Part model, mm, in its own coordinate system. Face numbers are marked on the shaded views. A direction names the side the tool comes from. Coordinates: 2 decimals unless noted, no trailing zeros. Order: outer loops, then holes, each group sorted by start corner. A loop starts at its lowest first (then second) coordinate and runs counter-clockwise, first axis right, second up.
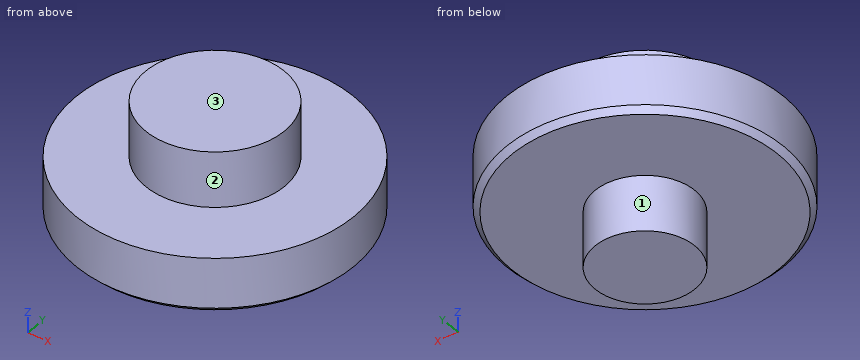
from build123d import *

# Parameters (mm, degrees)
SKETCH_R     = 50
PAD_DEPTH    = 20
CHAMFER_SIZE = 2
SKETCH001_R  = 18
PAD001_DEPTH = 20
SKETCH002_R  = 25
PAD002_DEPTH = 20


with BuildPart() as part:
    # Sketch → Pad (new body)
    with BuildSketch(Plane.XY):
        Circle(SKETCH_R)
    extrude(amount=PAD_DEPTH)

    # Chamfer
    chamfer_edges = [part.edges().sort_by_distance(p)[0] for p in [
        (-50, 0, 0),
    ]]
    chamfer(chamfer_edges, length=CHAMFER_SIZE)

    # Sketch001 (on Face4 of Chamfer) → Pad001 (join)
    with BuildSketch(Plane(origin=(0, 0, 0), x_dir=(1, 0, 0), z_dir=(0, 0, -1))):
        Circle(SKETCH001_R)
    extrude(amount=PAD001_DEPTH)

    # Sketch002 (on Face3 of Pad001) → Pad002 (join)
    with BuildSketch(Plane.XY.offset(20)):
        Circle(SKETCH002_R)
    extrude(amount=PAD002_DEPTH)


solid = part.part
Q1. Cut at D-D on z = -5. Write the cut outline in (x, y).
Results list:
outline: circle Ø36 at (0, 0)
Q2. Which spindle directions (+Z, -Z, +X, -X, +Y, -Y) get a long thin tool onto all of the face, cutting with end or side? Do the marked faces 1, 2 and 3. Say none if no direction does.
Results list:
face 1: -Z
face 2: +Z
face 3: +Z, +X, -X, +Y, -Y
Q3. Wall check: line 1 along Z through (x, y) = (39, -4); line 2 along Z through (x, y) = (-11, 21.5); line 3 along X through (y, z) = (-1.5, 7.5). Give the ranges that are in metal, low to high.
Results list:
line 1: z = 0 to 20
line 2: z = 0 to 40
line 3: x = -49.98 to 49.98
Q4. Cut at A-A on x = 0. Write the cut outline in (y, z).
Results list:
outline: (-50, 2) - (-48, 0) - (-18, 0) - (-18, -20) - (18, -20) - (18, 0) - (48, 0) - (50, 2) - (50, 20) - (25, 20) - (25, 40) - (-25, 40) - (-25, 20) - (-50, 20) - close
Q5. Cut at C-C on z = 12. Write the cut outline in (x, y).
Results list:
outline: circle Ø100 at (0, 0)
Q6. Pin check, flat tips, straight feed: pin 1 Ø4 at (y, z) = (16, 18.5) entering from +X; pin 2 Ø1.5 at (x, y) = (-14.5, -34.5) entering from -Z; pin 3 Ø2 at (x, z) = (14, -5.5) entering from +Y. Stop position of each tip, or through.
Results list:
pin 1: stops at x = 48
pin 2: stops at z = 0
pin 3: stops at y = 12.45
